Can you work these out from the model? Positions are in its coordinate system, mm. A direction names the side the tool comes from. Give positions to 0.01 mm unless a question says otherwise; leave off trailing zeros. Write each loop counter-clockwise with the first axis right and the second up, starting at its lowest first coordinate (ties: lowest second). Pieces come first, ordered by that corner, then holes.
1. Suppose I cut it at A-A (z = -38). Please give me the cut outline in (x, y).
2. I'm going to push a flat-ended pin straight in: pin 1 (2 mm diameter, centred on x = 5, z = 28, fed in from +Y). Where does the tip first touch, or does it pass through?
3. If I drill on probe 1 along X at (y, z) = (0.55, 31); probe 2 along X at (y, z) = (1.45, 18); probe 3 along Z at (x, y) = (-36.5, 1.45), over which ranges is the centre line in solid material (lowest first)?
4. Suppose I cut it at C-C (z = -8). Please give me the cut outline in (x, y), and give its area (3 significant figures).
5. On a 3-axis mill with a long thin cutter (end or side, diameter ignored), from which of +Z, -Z, +X, -X, +Y, -Y can I reach the whole of each face in a straight line? I mean faces 3 (the flat face through (-34, 3, -4)), 4 (the cylindrical face through (-100.68, 1.52, 41.61)), 5 (the flat face through (45, 1, 37)). Say none if no direction works.
6. Suppose I cut it at B-B (x = -40). Please give me the cut outline in (y, z), and give its area (3 significant figures).
7. Suppose I cut it at D-D (y = 2.1). Give the number of separate pieces and of enclosed holes in the cut face, and give its area (3 significant figures).
8. Thinking about a two-plate mould opening in X: for faces 1 (the cylindrical face through (-17.692, 1.521, -47.685)), 2 (the flat face through (-34, 0, -4)), which applies, pulls with the +X half, pulls with the -X half, needs draft (parallel to the pull), parting line crosses it, or undercut?
```python
from build123d import *

# Parameters (mm, degrees)
SKETCH_1_W          = 229
SKETCH_1_H          = 115
EXTRUDE_1_DEPTH     = 3
SKETCH_2_W          = 84
SKETCH_2_H          = 99.5
CUT_EXTRUDE_2_DEPTH = 2
SKETCH_4_W          = 78
SKETCH_4_H          = 96.5
CUT_EXTRUDE_3_DEPTH = 2
SKETCH_5_R          = 1.75
CUT_EXTRUDE_4_DEPTH = 3


with BuildPart() as part:
    # 草图1 → 凸台-拉伸1 (new body)
    with BuildSketch(Plane(origin=(0, 0, 0), x_dir=(1, 0, 0), z_dir=(0, 1, 0))):
        with Locations((-7.184913218, 3.036715621)):
            Rectangle(SKETCH_1_W, SKETCH_1_H)
    extrude(amount=EXTRUDE_1_DEPTH)

    # 草图2 → 切除-拉伸2 (cut)
    with BuildSketch(Plane(origin=(0, 3, 0), x_dir=(1, 0, 0), z_dir=(0, 1, 0))):
        with Locations((45.315086782, 10.786715621)):
            Rectangle(SKETCH_2_W, SKETCH_2_H)
    extrude(amount=-CUT_EXTRUDE_2_DEPTH, mode=Mode.SUBTRACT)

    # 草图4 → 切除-拉伸3 (cut)
    with BuildSketch(Plane(origin=(0, 1, 0), x_dir=(1, 0, 0), z_dir=(0, 1, 0))):
        with Locations((45.315086782, 12.286715621)):
            Rectangle(SKETCH_4_W, SKETCH_4_H)
    extrude(amount=-CUT_EXTRUDE_3_DEPTH, mode=Mode.SUBTRACT)

    # 草图5 → 切除-拉伸4 (cut)
    with BuildSketch(Plane(origin=(0, 3, 0), x_dir=(1, 0, 0), z_dir=(0, 1, 0))):
        with Locations(Location((-64.684913218, 3.036715621, 0), (0, 0, 270))):
            Circle(SKETCH_5_R)
        with Locations(Location((-24.684913218, 3.036715621, 0), (0, 0, 270))):
            Circle(SKETCH_5_R)
        with Locations(Location((-2.684913218, 54.536715621, 0), (0, 0, 270))):
            Circle(SKETCH_5_R)
        with Locations(Location((93.315086782, 54.536715621, 0), (0, 0, 270))):
            Circle(SKETCH_5_R)
        with Locations(Location((93.315086782, -32.963284379, 0), (0, 0, 270))):
            Circle(SKETCH_5_R)
        with Locations(Location((-2.684913218, -32.963284379, 0), (0, 0, 270))):
            Circle(SKETCH_5_R)
        with BuildLine():
            Line((-93.684913218, 50.536715621), (-24.684913218, 50.536715621))
            ThreePointArc((-24.684913218, 50.536715621), (-17.613845406, 47.607783433), (-14.684913218, 40.536715621))
            Line((-14.684913218, 40.536715621), (-14.684913218, 23.036715621))
            ThreePointArc((-14.684913218, 23.036715621), (-17.613845406, 15.965647809), (-24.684913218, 13.036715621))
            Line((-24.684913218, 13.036715621), (-93.684913218, 13.036715621))
            ThreePointArc((-93.684913218, 13.036715621), (-100.755981029, 15.965647809), (-103.684913218, 23.036715621))
            Line((-103.684913218, 23.036715621), (-103.684913218, 40.536715621))
            ThreePointArc((-103.684913218, 40.536715621), (-100.755981029, 47.607783433), (-93.684913218, 50.536715621))
        make_face()
        with BuildLine():
            Line((-93.684913218, -6.963284379), (-24.684913218, -6.963284379))
            ThreePointArc((-24.684913218, -6.963284379), (-17.613845406, -9.892216567), (-14.684913218, -16.963284379))
            Line((-14.684913218, -16.963284379), (-14.684913218, -34.463284379))
            ThreePointArc((-14.684913218, -34.463284379), (-17.613845406, -41.534352191), (-24.684913218, -44.463284379))
            Line((-24.684913218, -44.463284379), (-93.684913218, -44.463284379))
            ThreePointArc((-93.684913218, -44.463284379), (-100.755981029, -41.534352191), (-103.684913218, -34.463284379))
            Line((-103.684913218, -34.463284379), (-103.684913218, -16.963284379))
            ThreePointArc((-103.684913218, -16.963284379), (-100.755981029, -9.892216567), (-93.684913218, -6.963284379))
        make_face()
    extrude(amount=-CUT_EXTRUDE_4_DEPTH, mode=Mode.SUBTRACT)


solid = part.part
```
Checks:
1. outline: (-121.68, 0) - (-103.68, 0) - (-103.68, 3) - (-121.68, 3) - close; (-14.68, 0) - (6.32, 0) - (6.32, 1) - (3.32, 1) - (3.32, 3) - (-14.68, 3) - close; (84.32, 0) - (107.32, 0) - (107.32, 3) - (87.32, 3) - (87.32, 1) - (84.32, 1) - close
2. pin 1: stops at y = 1
3. probe 1: x = -121.68 to -103.68, -14.68 to 6.32, 84.32 to 107.32
3. probe 2: x = -121.68 to -103.68, -14.68 to 3.32, 87.32 to 107.32
3. probe 3: z = -60.54 to -50.54, -13.04 to 6.96, 44.46 to 54.46
4. outline: (-121.68, 0) - (6.32, 0) - (6.32, 1) - (3.32, 1) - (3.32, 3) - (-121.68, 3) - close; (84.32, 0) - (107.32, 0) - (107.32, 3) - (87.32, 3) - (87.32, 1) - (84.32, 1) - close
4. area: 441 mm2
5. face 3: +Z, -Z, +X, -X, +Y
5. face 4: +Y, -Y
5. face 5: -Z, +Y
6. outline: (0, -60.54) - (3, -60.54) - (3, -50.54) - (0, -50.54) - close; (0, -13.04) - (3, -13.04) - (3, 6.96) - (0, 6.96) - close; (0, 44.46) - (3, 44.46) - (3, 54.46) - (0, 54.46) - close
6. area: 120 mm2
7. separate pieces: 1
7. enclosed holes: 8
7. area: 11,400 mm2
8. face 1: undercut
8. face 2: needs draft
